```python
from build123d import *

# Parameters (mm, degrees)
F0_W     = 50.6739839911
F0_H     = 37.3927876353
F1_DEPTH = 800
F2_DEPTH = 600
F3_DEPTH = 600
F4_T     = -18


with BuildPart() as f1:
    # F0 (on Top) → F1 (new body)
    with BuildSketch(Plane.XY):
        with Locations((25.3369919956, -18.6963938177)):
            Rectangle(F0_W, F0_H)
    extrude(amount=F1_DEPTH)

    # F2 (add): a face of the model
    f2_faces = [f1.faces().sort_by_distance(p)[0] for p in [
        (0, -18.6963938177, 400),
    ]]
    extrude(f2_faces, amount=-F2_DEPTH)

    # F3 (add): a face of the model
    f3_faces = [f1.faces().sort_by_distance(p)[0] for p in [
        (300, 0, 400),
    ]]
    extrude(f3_faces, amount=-F3_DEPTH)

    # F4
    f4_openings = [f1.faces().sort_by_distance(p)[0] for p in [
        (300, -600, 400),
    ]]
    offset(amount=F4_T, openings=f4_openings)


solid = f1.part
```
Build history of the part. All positions in model axes, mm. A direction names the side the tool comes from. Round coordinates to 2 decimals unless told otherwise and drop trailing zeros. Write each loop counter-clockwise with the first axis right and the second up, starting at its lowest first coordinate (ties: lowest second). Pieces come first, ordered by that corner, then holes.
1) 3-axis set-ups, long thin cutter, end or side, ignore diameter. For faces 4 (the flat face through (18, -305, 395)), 5 (the flat face through (10, -600, 398)): which of +Z, -Z, +X, -X, +Y, -Y reach the whole face in a straight line?
2) Mould opens along X. For faces 1 (the flat face through (296, 0, 394)), 2 (the flat face through (296, -18, 395)), 3 (the flat face through (0, -296, 394)) say: +X half, -X half, draft (parallel to the pull), parting line (faces both ways), or undercut.
3) Pin check, flat tip, straight feed: pin 1 (4 mm diameter, centred on x = 230.5, z = 474.5, fed in from -Y). Stop position of the tip, or through.
4) Band-saw the part on C-C, the plane x = 328.5. List the corners of the cut face in (y, z), and give its area (3 significant figures).
5) Band-saw the part on A-A, the plane y = -72. List the corners of the cut face in (x, z), and give its area (3 significant figures).
6) Band-saw the part on B-B, the plane z = 427.5. List the corners of the cut face in (x, y), and give its area (3 significant figures).
7) Drill centre lines: probe 1 along Z at (x, y) = (100, -283.5); probe 2 along X at (y, z) = (-200.5, 290.5); probe 3 along Y at (x, z) = (320, 565). Where is each one in solid material? Low to high.
Ans:
1. face 4: -Y
1. face 5: +Z, -Z, +X, -X, -Y
2. face 1: draft
2. face 2: undercut
2. face 3: -X half
3. pin 1: stops at y = -18
4. outline: (-600, 0) - (0, 0) - (0, 800) - (-600, 800) - (-600, 782) - (-18, 782) - (-18, 18) - (-600, 18) - close
4. area: 35,400 mm2
5. outline: (0, 0) - (600, 0) - (600, 800) - (0, 800) - close; hole (18, 18) - (582, 18) - (582, 782) - (18, 782) - close
5. area: 49,100 mm2
6. outline: (0, -600) - (18, -600) - (18, -18) - (582, -18) - (582, -600) - (600, -600) - (600, 0) - (0, 0) - close
6. area: 31,800 mm2
7. probe 1: z = 0 to 18, 782 to 800
7. probe 2: x = 0 to 18, 582 to 600
7. probe 3: y = -18 to 0
